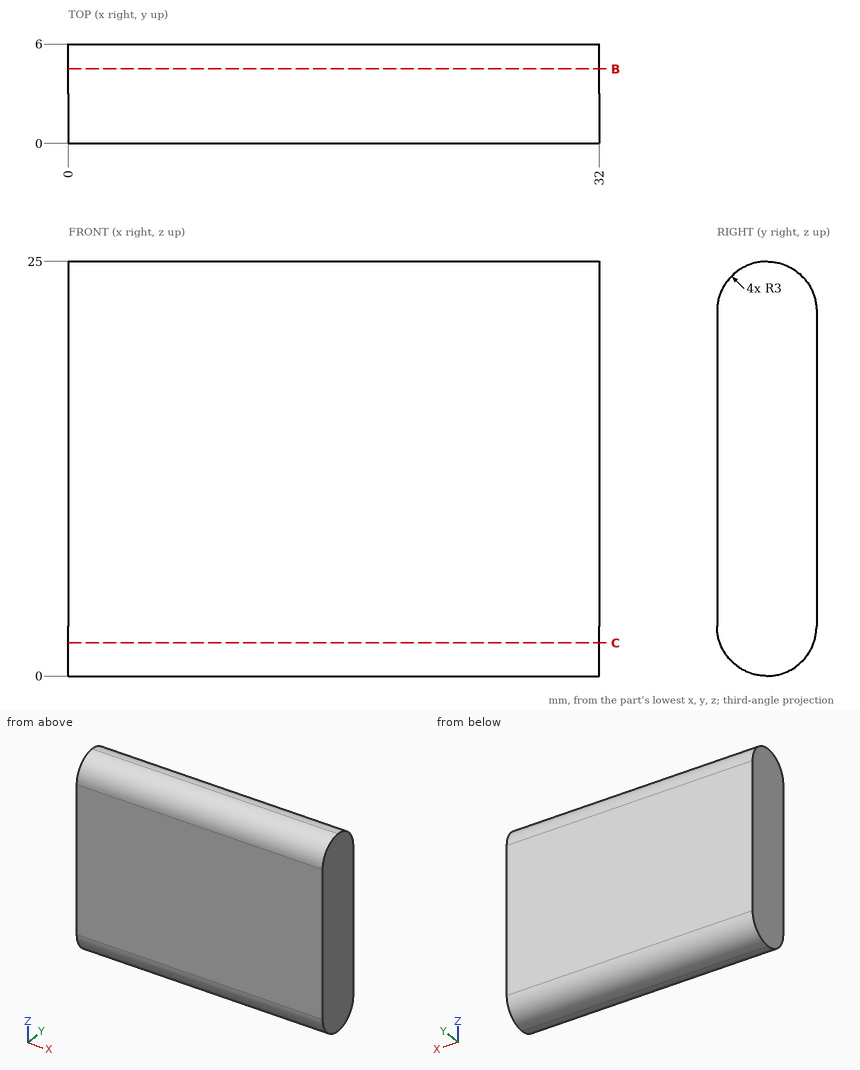
Design review of the part shown in the three views and the two pictorial views. Dimensions are in mm from the part's minimum x, y and z. Give positions to 0.01 mm unless a question says otherwise; leave off trailing zeros. Write each loop counter-clockwise with the first axis right and the second up, starting at its lowest first coordinate (ties: lowest second). Pieces come first, ordered by that corner, then holes. Notation, with made-up numbers: M -27.5,27 L -5.5,27 A22 ccw -5.5,61 Z; hole C 37.5,-19 d8. An arc over 180 degrees is marked long. Answer in a Markdown table with one row per item.
Item 1: Add section C-C on z = 2. Give the boundary of the cut face in (x, y).
Check sheet entries:
| item | result |
|---|---|
| outline | M 0,0.17 L 32,0.17 L 32,5.83 L 0,5.83 Z |
Item 2: Add section B-B on y = 4.5. Give the boundary of the cut face in (x, z), plus the area to 3 significant figures.
Check sheet entries:
| item | result |
|---|---|
| outline | M 0,0.4 L 32,0.4 L 32,24.6 L 0,24.6 Z |
| area | 774 mm2 |
Item 3: For line 1 along Z through (x, y) = (9, 5.5); line 2 along Z through (x, y) = (6, 1.25), list the stretches that pass through material, from the lowest coordinate up.
Check sheet entries:
| item | result |
|---|---|
| line 1 | 1.34 to 23.66 |
| line 2 | 0.56 to 24.44 |
Item 4: For P1, Ø1, axis at x = 24, y = 1, coming from the -Z side; P2, Ø2, axis at x = 28, y = 5, coming from the -Z side; P3, Ø1.5, axis at x = 8, y = 4.5, coming from the +Z side, all flat-tipped, find the tip position at first contact; note any pin that passes through.
Check sheet entries:
| item | result |
|---|---|
| P1 | z = 0.4 |
| P2 | z = 0.17 |
| P3 | z = 24.9 |
